Input: part model. Units: mm. Frame: model coordinates. A direction names the side the tool comes from. Coordinates: 2 decimals unless noted, no trailing zeros. Order: outer loops, then holes, each group sorted by start corner. A loop starts at its lowest first (then second) coordinate and runs counter-clockwise, first axis right, second up. Notation, with made-up numbers: M -28,-25.5 L -5,-25.5 A33 ccw -5,11.5 Z; hole C 70.5,-26.5 d7. An arc over 180 degrees is marked long. One line per item, written item: value.
```python
from build123d import *

# Parameters (mm, degrees)
BOSS_EXTRUDE1_DEPTH = 42.4
SKETCH3_R           = 11
SKETCH3_R_2         = 1.5
CUT_EXTRUDE1_DEPTH  = 7


with BuildPart() as part:
    # Sketch2 → Boss-Extrude1 (new body)
    with BuildSketch(Plane(origin=(0, 0, 0), x_dir=(1, 0, 0), z_dir=(0, 1, 0))):
        Polygon((-42.4, 0), (0, 0), (0, -30), (6, -30), (6, 6), (-42.4, 6), align=None)
    extrude(amount=BOSS_EXTRUDE1_DEPTH)

    # Sketch3 → Cut-Extrude1 (cut, through all)
    with BuildSketch(Plane.XY):
        with Locations((-21.2, 21.2)):
            Circle(SKETCH3_R)
        with Locations((-36.7, 36.7)):
            Circle(SKETCH3_R_2)
        with Locations((-5.7, 36.7)):
            Circle(SKETCH3_R_2)
        with Locations((-5.7, 5.7)):
            Circle(SKETCH3_R_2)
        with Locations((-36.7, 5.7)):
            Circle(SKETCH3_R_2)
    extrude(amount=-CUT_EXTRUDE1_DEPTH, mode=Mode.SUBTRACT)


solid = part.part
```
(1) Draft query along Y for faces 3 (the flat face through (-12, 11, 0)), 4 (the cylindrical face through (-35.314, 5.125, -2.958)), 5 (the flat face through (-15, 0, -1)), 6 (the cylindrical face through (-32.19, 21.68, -2.96)). Return one class per face: released by +Y, released by -Y, zero draft, split by the parting line, or undercut.
Data:
face 3: zero draft
face 4: undercut
face 5: released by -Y
face 6: undercut
(2) Cut plane C-C on x = -29.5. Output: boundary loops of the cut face in (y, z), plus the area to 3 significant figures.
Data:
outline: M 0,-6 L 13.98,-6 L 13.98,0 L 0,0 Z; M 28.42,-6 L 42.4,-6 L 42.4,0 L 28.42,0 Z
area: 168 mm2
(3) Cut plane A-A on y = 21.2. Output: boundary loops of the cut face in (x, z), plus the area to 3 significant figures.
Data:
outline: M -42.4,-6 L -32.2,-6 L -32.2,0 L -42.4,0 Z; M -10.2,-6 L 6,-6 L 6,30 L 0,30 L 0,0 L -10.2,0 Z
area: 338 mm2
(4) Cut plane D-D on y = 36.7. Output: boundary loops of the cut face in (x, z), plus the area to 3 significant figures.
Data:
outline: M -42.4,-6 L -38.2,-6 L -38.2,0 L -42.4,0 Z; M -35.2,-6 L -7.2,-6 L -7.2,0 L -35.2,0 Z; M -4.2,-6 L 6,-6 L 6,30 L 0,30 L 0,0 L -4.2,0 Z
area: 434 mm2
(5) Cut plane B-B on x = -5.7. Output: boundary loops of the cut face in (y, z), plus the area to 3 significant figures.
Data:
outline: M 0,-6 L 4.2,-6 L 4.2,0 L 0,0 Z; M 7.2,-6 L 35.2,-6 L 35.2,0 L 7.2,0 Z; M 38.2,-6 L 42.4,-6 L 42.4,0 L 38.2,0 Z
area: 218 mm2
(6) Access query for faces 1 (the flat face through (0, 21, 15)), 2 (the cylindrical face through (-6.9, 4.8, -3)). Directions: +Z, -Z, +X, -X, +Y, -Y. A direction counts if a zero-diameter tool reaches every point of the face in a straight line with its end or side. Return the directions, or none.
Data:
face 1: +Z, -X, +Y, -Y
face 2: +Z, -Z
(7) Ray query, line 1 (Y direction, x = -36.7, z = -4.55); line 2 (X direction, y = 21, z = -3); line 3 (X direction, y = 36, z = -3). Return the intervals inside material, ascending. Write a range as from..to.
Data:
line 1: y = 0..4.2, 7.2..35.2, 38.2..42.4
line 2: x = -42.4..-32.2, -10.2..6
line 3: x = -42.4..-38.03, -35.37..-7.03, -4.37..6
(8) First-contact query: pin 1 (1 mm diameter, centred on x = -35.5, y = 36, fed in from +Z); pin 2 (13 mm diameter, centred on x = -21.2, y = 21.2, fed in from +Z); pin 3 (4 mm diameter, centred on y = 21, z = 4, fed in from -X). Flat tips, straight axial feed; report the tip coordinate or a pass-through.
Data:
pin 1: stops at z = 0
pin 2: passes through
pin 3: stops at x = 0
